Part print with two shaded views. Sizes in mm from the minimum x, y, z corner. A direction names the side the tool comes from. Coordinates: 2 decimals unless noted, no trailing zeros. Order: outer loops, then holes, each group sorted by start corner. A loop starts at its lowest first (then second) coordinate and runs counter-clockwise, first axis right, second up.
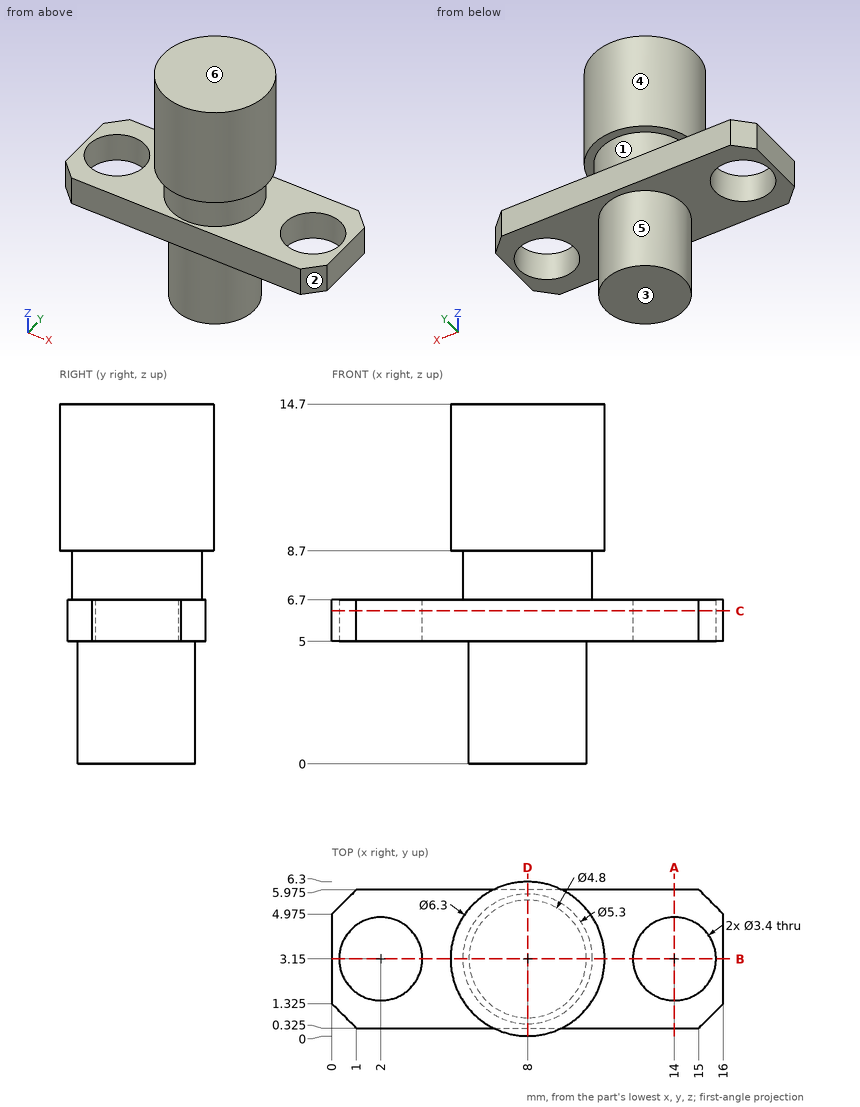
Q1. Mould opens along Z. For the marked faces 1, 2 and 3 say: pulls with the +Z half, pulls with the -Z half, needs draft (parallel to the pull), parting line crosses it, or undercut.
Results list:
face 1: undercut
face 2: needs draft
face 3: pulls with the -Z half
Q2. Pin check, flat tips, straight feed: pin 1 Ø2.5 at (x, y) = (14, 3.15) entering from +Z; pin 2 Ø2 at (y, z) = (1, 13) entering from +X; pin 3 Ø1.9 at (x, z) = (9.5, 6) entering from +Y (3 decimals); pin 4 Ø1.4 at (x, z) = (6, 5.5) entering from -Y (3 decimals). Stop position of each tip, or through.
Results list:
pin 1: passes through
pin 2: stops at x = 10.93
pin 3: stops at y = 5.975
pin 4: stops at y = 0.325
Q3. Wall check: line 1 along Y through (x, z) = (2, 5.9) (3 decimals); line 2 along Z through (x, y) = (7.25, 0.5); line 3 along X through (y, z) = (3, 12.5). Give the ranges that are in metal, low to high.
Results list:
line 1: y = 0.325 to 1.45, 4.85 to 5.975
line 2: z = 5 to 6.7, 8.7 to 14.7
line 3: x = 4.85 to 11.15
Q4. Cut at D-D on x = 8. Write the cut outline in (y, z) (3 decimals).
Results list:
outline: (0, 8.7) - (0.5, 8.7) - (0.5, 6.7) - (0.325, 6.7) - (0.325, 5) - (0.75, 5) - (0.75, 0) - (5.55, 0) - (5.55, 5) - (5.975, 5) - (5.975, 6.7) - (5.8, 6.7) - (5.8, 8.7) - (6.3, 8.7) - (6.3, 14.7) - (0, 14.7) - close
Q5. Which spindle directions (+Z, -Z, +X, -X, +Y, -Y) get a long thin tool onto all of the face, cutting with end or side? Do the marked faces 4, 5 and 6. Say none if no direction does.
Results list:
face 4: +Z
face 5: -Z
face 6: +Z, +X, -X, +Y, -Y
Q6. Cut at B-B on y = 3.15. Write the cut outline in (x, z).
Results list:
outline: (0, 5) - (0.3, 5) - (0.3, 6.7) - (0, 6.7) - close; (3.7, 5) - (5.6, 5) - (5.6, 0) - (10.4, 0) - (10.4, 5) - (12.3, 5) - (12.3, 6.7) - (10.65, 6.7) - (10.65, 8.7) - (11.15, 8.7) - (11.15, 14.7) - (4.85, 14.7) - (4.85, 8.7) - (5.35, 8.7) - (5.35, 6.7) - (3.7, 6.7) - close; (15.7, 5) - (16, 5) - (16, 6.7) - (15.7, 6.7) - close
Q7. Cut at A-A on x = 14. Write the cut outline in (y, z) (3 decimals).
Results list:
outline: (0.325, 5) - (1.45, 5) - (1.45, 6.7) - (0.325, 6.7) - close; (4.85, 5) - (5.975, 5) - (5.975, 6.7) - (4.85, 6.7) - close
Q8. Cut at C-C on z = 6.25. Write the cut outline in (x, y) (3 decimals).
Results list:
outline: (0, 1.325) - (1, 0.325) - (15, 0.325) - (16, 1.325) - (16, 4.975) - (15, 5.975) - (1, 5.975) - (0, 4.975) - close; hole circle Ø3.4 at (2, 3.15); hole circle Ø3.4 at (14, 3.15)
